Here's how the part is built. I have some questions about the finished solid (model axes, mm). A direction names the side the tool comes from. Round coordinates to 2 decimals unless told otherwise and drop trailing zeros. Order: outer loops, then holes, each group sorted by start corner. A loop starts at its lowest first (then second) coordinate and runs counter-clockwise, first axis right, second up. Notation, with made-up numbers: (46, 61) -> (52, 61) arc R12 ccw to (52, 68) -> close; hole circle Ø10 at (4.25, 82). An arc over 180 degrees is marked (long way). Use a Markdown table: item, result. Add a question column.
(1) I'm going to push flat-ended pins straight in: P1, Ø1.5, axis at x = -334, z = 1.5, coming from the +Y side; P2, Ø1.5, axis at x = -369, z = 0.5, coming from the +Y side. Where does each tip first touch, or does it pass through?
(2) I want a section at A-A, the plane y = -98. Please give me the cut outline in (x, z).
(3) If I drill on probe 1 along X at (y, z) = (-81.5, 1.7); probe 2 along X at (y, z) = (-70, 0.25); probe 3 along Y at (x, z) = (-326.5, 2.5), over which ranges is the centre line in solid material (lowest first)?
(4) Thinking about a two-plate mould opening in Y: for faces 1 (the face through (-348.598, -42.084, 1.521)), 2 (the face through (-359.47, -103.48, 1.48)), 3 (the face through (-400.81, -34.92, 1.52)), which applies, pulls with the +Y half, pulls with the -Y half, needs draft (parallel to the pull), parting line crosses it, or undercut?
(5) I want a section at D-D, the plane y = -23.5. Please give me the cut outline in (x, z), then the cut area to 3 significant figures.
(6) I want a section at C-C, the plane z = 1.65. Please give me the cut outline in (x, y).
(7) I want a section at B-B, the plane x = -312. Please give me the cut outline in (y, z), then the cut area to 3 significant figures.
(8) On a 3-axis mill with a long thin cutter (end or side, diameter ignored), from which of +Z, -Z, +X, -X, +Y, -Y can I reach the whole of each face in a straight line? I mean faces 4 (the face through (-394.384, -57.783, 1.521)), 5 (the face through (-348.066, -92.392, 1.521)). Say none if no direction works.
from build123d import *

# Parameters (mm, degrees)
SKETCH_1_R         = 4.5
SKETCH_1_R_2       = 1.6
EXTRUDE_1_DEPTH    = 3
CUT_EXTRUDE1_DEPTH = 3


with BuildPart() as part:
    # 草图1 → 凸台-拉伸1 (new body)
    with BuildSketch(Plane.XY):
        Polygon((-329.573940975, -130.885149725), (-282.274763971, -79.282941877), (-355.992203754, -11.712689014), (-384.249742283, -12.942126399), (-404.520818142, -35.057358334), (-403.291380758, -63.314896863), align=None)
        with Locations((-383.327664245, -34.135280295)):
            Circle(SKETCH_1_R, mode=Mode.SUBTRACT)
        with Locations((-333.628644179, -119.029375523)):
            Circle(SKETCH_1_R_2, mode=Mode.SUBTRACT)
        with Locations((-325.520213836, -110.183282749)):
            Circle(SKETCH_1_R_2, mode=Mode.SUBTRACT)
        with Locations((-302.546327862, -85.119353223)):
            Circle(SKETCH_1_R_2, mode=Mode.SUBTRACT)
        with Locations((-294.437897519, -76.273260449)):
            Circle(SKETCH_1_R_2, mode=Mode.SUBTRACT)
    extrude(amount=EXTRUDE_1_DEPTH)

    # Sketch1 → Cut-Extrude1 (cut)
    with BuildSketch(Plane.XY.offset(3)):
        with BuildLine():
            Line((-400.059680241, -39.262622756), (-388.547892801, -76.828947435))
            Line((-388.547892801, -76.828947435), (-464.128258323, -22.526868134))
            Line((-464.128258323, -22.526868134), (-423.376063206, 22.684533744))
            Line((-423.376063206, 22.684533744), (-334.935129122, 6.829576373))
            Line((-334.935129122, 6.829576373), (-341.248715798, -25.226739587))
            Line((-341.248715798, -25.226739587), (-379.672909098, -17.021170187))
            ThreePointArc((-379.672909098, -17.021170187), (-396.228216207, -22.310486045), (-400.059680241, -39.262622756))
        make_face()
        with BuildLine():
            Line((-373.620721286, -70.163397904), (-349.668317732, -92.118446391))
            ThreePointArc((-349.668317732, -92.118446391), (-348.043488399, -92.382481208), (-347.154848014, -90.996803392))
            Line((-347.154848014, -90.996803392), (-347.658183177, -43.459413358))
            ThreePointArc((-347.658183177, -43.459413358), (-348.621743848, -42.074465348), (-350.263860698, -42.461740967))
            Line((-350.263860698, -42.461740967), (-373.71292909, -68.044082514))
            ThreePointArc((-373.71292909, -68.044082514), (-374.105749776, -69.12283707), (-373.620721286, -70.163397904))
        make_face()
        with BuildLine():
            Line((-330.000431814, -55.885012577), (-306.04802826, -77.840061064))
            ThreePointArc((-306.04802826, -77.840061064), (-305.56299977, -78.880621898), (-305.955820457, -79.959376454))
            Line((-305.955820457, -79.959376454), (-329.404888848, -105.541718001))
            ThreePointArc((-329.404888848, -105.541718001), (-331.047005699, -105.92899362), (-332.010566369, -104.544045611))
            Line((-332.010566369, -104.544045611), (-332.513901532, -57.006655576))
            ThreePointArc((-332.513901532, -57.006655576), (-331.625261147, -55.62097776), (-330.000431814, -55.885012577))
        make_face()
    extrude(amount=-CUT_EXTRUDE1_DEPTH, mode=Mode.SUBTRACT)


solid = part.part
Taken from the geometry:
| question | item | result |
|---|---|---|
| 1 | P1 | stops at y = -31.18 |
| 1 | P2 | stops at y = -19.14 |
| 2 | outline | (-365.45, 0) -> (-332.08, 0) -> (-332.08, 3) -> (-365.45, 3) -> close; (-322.49, 0) -> (-299.43, 0) -> (-299.43, 3) -> (-322.49, 3) -> close |
| 3 | probe 1 | x = -383.45 to -361.25, -347.26 to -332.25, -307.37 to -284.31 |
| 3 | probe 2 | x = -390.64 to -373.77, -347.38 to -332.38, -314.6 to -292.4 |
| 3 | probe 3 | y = -127.53 to -111.45, -108.92 to -102.37, -59.09 to -38.75 |
| 4 | face 1 | undercut |
| 4 | face 2 | pulls with the -Y half |
| 4 | face 3 | parting line crosses it |
| 5 | outline | (-393.93, 0) -> (-349.33, 0) -> (-349.33, 3) -> (-393.93, 3) -> close |
| 5 | area | 134 mm2 |
| 6 | outline | (-400.48, -30.64) arc R17.5 ccw to (-400.06, -39.26) -> (-388.55, -76.83) -> (-329.57, -130.89) -> (-282.27, -79.28) -> (-341.25, -25.23) -> (-379.67, -17.02) arc R17.5 ccw to (-388.29, -17.35) -> close; hole circle Ø9 at (-383.33, -34.14); hole (-373.71, -68.04) arc R1.5 ccw to (-373.62, -70.16) -> (-349.67, -92.12) arc R1.5 ccw to (-347.15, -91) -> (-347.66, -43.46) arc R1.5 ccw to (-350.26, -42.46) -> close; hole circle Ø3.2 at (-333.63, -119.03); hole (-332.51, -57.01) -> (-332.01, -104.54) arc R1.5 ccw to (-329.4, -105.54) -> (-305.96, -79.96) arc R1.5 ccw to (-306.05, -77.84) -> (-330, -55.89) arc R1.5 ccw to start; hole circle Ø3.2 at (-325.52, -110.18); hole circle Ø3.2 at (-302.55, -85.12); hole circle Ø3.2 at (-294.44, -76.27) |
| 7 | outline | (-111.71, 0) -> (-86.55, 0) -> (-86.55, 3) -> (-111.71, 3) -> close; (-72.38, 0) -> (-52.04, 0) -> (-52.04, 3) -> (-72.38, 3) -> close |
| 7 | area | 137 mm2 |
| 8 | face 4 | +Z, -Z, -X, -Y |
| 8 | face 5 | +Z, -Z |
